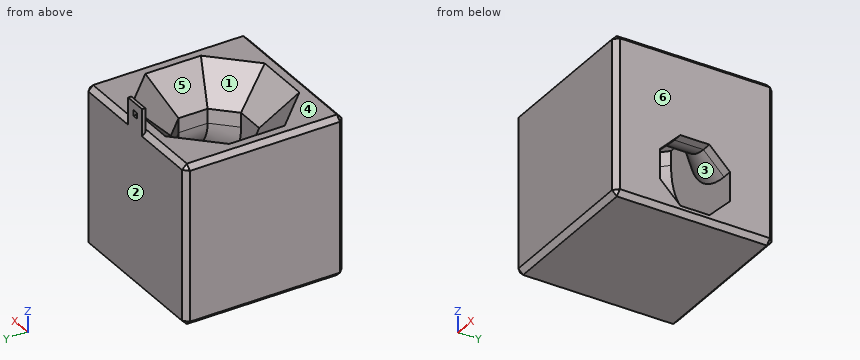
from build123d import *

# Parameters (mm, degrees)
SKETCH1_W                = 50
SKETCH1_H                = 50
BOSS_EXTRUDE1_DEPTH      = 50
CHAMFER1_SIZE            = 10
CHAMFER2_SIZE            = 1.5
BOSS_EXTRUDE2_DEPTH      = 7
BOSS_EXTRUDE2_DEPTH_BACK = 10
SKETCH10_W               = 7
SKETCH10_H               = 1
SKETCH11_W               = 1.8
SKETCH11_H               = 1.8
CUT_EXTRUDE1_DEPTH       = 7


with BuildPart() as part:
    # Sketch1 → Boss-Extrude1 (new body)
    with BuildSketch(Plane.XY):
        with Locations((25, 25)):
            Rectangle(SKETCH1_W, SKETCH1_H)
    extrude(amount=BOSS_EXTRUDE1_DEPTH)

    # Cut-Sweep5: sweep along a path in Sketch9
    with BuildLine(Plane(origin=(0, 25, 0), x_dir=(-1, 0, 0), z_dir=(0, -1, 0))) as cut_sweep5_path:
        Line((-50, -13.5), (-47, -13.5))
        ThreePointArc((-47, -13.5), (-31.443650814, -19.943650814), (-25, -35.5))
        Line((-25, -35.5), (-25, -50))
    # Sketch8 → Cut-Sweep5 (sweep, cut)
    with BuildSketch(Plane(origin=(50, 0, 0), x_dir=(0, 0, -1), z_dir=(1, 0, 0))):
        Polygon((-2.5, 29.556349186), (-8.943650814, 36), (-18.056349186, 36), (-24.5, 29.556349186), (-24.5, 20.443650814), (-18.056349186, 14), (-8.943650814, 14), (-2.5, 20.443650814), align=None)
    sweep(path=cut_sweep5_path.line, mode=Mode.SUBTRACT)

    # Chamfer1
    chamfer1_edges = [part.edges().sort_by_distance(p)[0] for p in [
        (17.221825407, 17.221825407, 50),
        (32.778174593, 17.221825407, 50),
        (36, 25, 50),
        (32.778174593, 32.778174593, 50),
        (17.221825407, 32.778174593, 50),
        (14, 25, 50),
        (25, 14, 50),
        (25, 36, 50),
    ]]
    chamfer(chamfer1_edges, length=CHAMFER1_SIZE)

    # Chamfer2
    chamfer2_edges = [part.edges().sort_by_distance(p)[0] for p in [
        (50, 25, 50),
        (25, 50, 50),
        (0, 25, 50),
        (25, 50, 0),
        (50, 25, 0),
        (25, 0, 0),
        (0, 25, 0),
        (25, 0, 50),
        (0, 50, 25),
        (50, 50, 25),
        (50, 0, 25),
        (0, 0, 25),
    ]]
    chamfer(chamfer2_edges, length=CHAMFER2_SIZE)

    # Sketch10 → Boss-Extrude2 (add, two sides: drawn at the far end of the back side and taken through both)
    with BuildSketch(Plane.XY.offset(50).offset(-BOSS_EXTRUDE2_DEPTH_BACK)):
        with Locations((25, 49.5)):
            Rectangle(SKETCH10_W, SKETCH10_H)
    extrude(amount=BOSS_EXTRUDE2_DEPTH + BOSS_EXTRUDE2_DEPTH_BACK)

    # Sketch11 → Cut-Extrude1 (cut)
    with BuildSketch(Plane.XZ.offset(-49)):
        with Locations((25, 53.6)):
            Rectangle(SKETCH11_W, SKETCH11_H)
    extrude(amount=-CUT_EXTRUDE1_DEPTH, mode=Mode.SUBTRACT)


solid = part.part
Can you work these out from the model? Positions are in its coordinate system, mm. Face numbers are marked on the shaded views. A direction names the side the tool comes from. Coordinates: 2 decimals unless noted, no trailing zeros. Write each loop counter-clockwise with the first axis right and the second up, starting at its lowest first coordinate (ties: lowest second). Pieces come first, ordered by that corner, then holes.
Q1. If we mould it in two halves opening along X, with no side actions, what happens to the marked faces 4, 5 and 6? For each: +X half, -X half, draft (parallel to the pull), parting line (faces both ways), or undercut.
Results found:
face 4: draft
face 5: undercut
face 6: +X half
Q2. Imagine slicing it at C-C, the plane x = 8. List the corners of the cut face in (y, z) for me, plus the area to 3 significant figures.
Results found:
outline: (0, 1.5) - (1.5, 0) - (48.5, 0) - (50, 1.5) - (50, 48.5) - (48.5, 50) - (37.7, 50) - (32.04, 46) - (17.96, 46) - (12.3, 50) - (1.5, 50) - (0, 48.5) - close
area: 2,420 mm2
Q3. Imagine slicing it at B-B, the plane y = 6. List the corners of the cut face in (x, z) for me.
Results found:
outline: (0, 1.5) - (1.5, 0) - (48.5, 0) - (50, 1.5) - (50, 48.5) - (48.5, 50) - (35.7, 50) - (32.87, 48) - (17.13, 48) - (14.3, 50) - (1.5, 50) - (0, 48.5) - close
Q4. Which directions (+Z, -Z, +X, -X, +Y, -Y) give clear straight access to the entire face, cutting with the end or side of a thin tool? Please do the marked faces 1, 2 and 3.
Results found:
face 1: +Z
face 2: +Z, -Z, +X, -X, +Y
face 3: none
Q5. Imagine slicing it at D-D, the plane z = 47.5. List the corners of the cut face in (x, y) for me, plus the area to 3 significant figures.
Results found:
outline: (0, 1.5) - (1.5, 0) - (48.5, 0) - (50, 1.5) - (50, 48.5) - (48.5, 50) - (1.5, 50) - (0, 48.5) - close; hole (6.5, 17.34) - (17.34, 6.5) - (32.66, 6.5) - (43.5, 17.34) - (43.5, 32.66) - (32.66, 43.5) - (17.34, 43.5) - (6.5, 32.66) - close
area: 1,360 mm2
Q6. Imagine slicing it at A-A, the plane z = 37.5. List the corners of the cut face in (x, y) for me, plus the area to 3 significant figures.
Results found:
outline: (0, 1.5) - (1.5, 0) - (48.5, 0) - (50, 1.5) - (50, 48.5) - (48.5, 50) - (1.5, 50) - (0, 48.5) - close; hole (14, 20.44) - (20.44, 14) - (29.56, 14) - (36, 20.44) - (36, 29.56) - (29.56, 36) - (20.44, 36) - (14, 29.56) - close
area: 2,090 mm2
Q7. For P1, Ø3.5, axis at x = 49, y = 27, coming from the -Z side; P2, Ø0.8, axis at y = 49.5, z = 52.5, coming from the -X side; P3, Ø23.5, axis at x = 16, y = 24, coming from the +Z side; P4, Ø1.5, axis at x = 48.5, y = 25.5, coming from the +Z side, each with a flat end and sliding along its axis, tell me the tip position at first contact or that it passes through.
Results found:
P1: stops at z = 0
P2: stops at x = 21.5
P3: stops at z = 49.75
P4: stops at z = 50
Q8. Please list where these lines run through material, in increasing order: L1, parallel to Z at x = 46.5, y = 23; L2, parallel to Z at x = 4.5, y = 14; L3, parallel to X at y = 18, z = 27.
Results found:
L1: z = 0 to 2.5, 24.51 to 50
L2: z = 0 to 50
L3: x = 0 to 17.65, 36.58 to 50
